Design review of the part built by this model. Coordinates are the model's own, in mm. A direction names the side the tool comes from. Coordinates: 2 decimals unless noted, no trailing zeros. Loops run counter-clockwise (first coordinate to the right, second up) from the corner with the lowest first, then second, coordinate; pieces in that order, holes last.
from build123d import *

# Parameters (mm, degrees)
F1_DEPTH = 130


with BuildPart() as f1:
    # F0 (on Front) → F1 (new body)
    with BuildSketch(Plane.XZ):
        with BuildLine():
            Line((-80.4885666445, 0), (-80.4885666445, -37.026398866))
            Line((-80.4885666445, -37.026398866), (80.4885666445, -37.026398866))
            Line((80.4885666445, -37.026398866), (80.4885666445, 37.026398866))
            ThreePointArc((80.4885666445, 37.026398866), (56.312606492, 15.964739969), (24.5885544515, 11.3112416162))
            ThreePointArc((24.5885544515, 11.3112416162), (23.4644064233, 5.2103284523), (20.0973115861, 0))
            ThreePointArc((20.0973115861, 0), (10.0486557931, -1.628361225), (0, 0))
            add(Edge.make_bspline(
                [(0, 0), (1.1070352702, -1.6801785988), (3.1184613885, -4.7329766513), (4.5940239288, -8.7749202813), (1.7421748157, -13.92092092), (0, -17.0645769686)],
                knots=[0, 0, 0, 0, 0.3226277316, 0.5861979859, 1, 1, 1, 1], degree=3))
            Line((0, -17.0645769686), (-68.7817037106, -17.0645769686))
            add(Edge.make_bspline(
                [(-69.5971027017, 0), (-68.7549732227, -1.0893751099), (-72.5978419161, -5.9254448151), (-70.4120398181, -12.0907470214), (-69.2717425761, -15.6012676406), (-68.7817037106, -17.0645769686)],
                knots=[0.3125236167, 0.3125236167, 0.3125236167, 0.3125236167, 0.5421460101, 0.7849492257, 1, 1, 1, 1], degree=3))
            Line((-69.5971027017, 0), (-80.4885666445, 0))
        make_face()
    extrude(amount=F1_DEPTH)


solid = f1.part
Q1. For line 1 (X direction, y = -21.5, z = -4.5); line 2 (Z direction, x = -50, y = -68.5); line 3 (Z direction, x = 31, y = -91.5), list the stretches that pass through material, from the lowest coordinate up.
Q2. The part is to be moulded in two halves that separate along X. For faces 1 (the cylindrical face through (56.73, -64.09, 16.16)), 2 (the flat face through (17, -130, -16)), 3 (the flat face through (-80.489, -64, -18)), 4 (the flat face through (80.489, -64, -1)), say which applies: pulls with the +X half, pulls with the -X half, needs draft (parallel to the pull), parting line crosses it, or undercut.
Q3. Machinability: for faces 5 (the flat face through (-1, -64, -37.026)), 6 (the flat face through (-34, -64, -17.065)), 7 (the flat face through (-75, -64, 0)), which of the approach directions +Z, -Z, +X, -X, +Y, -Y give a long, thin tool a straight path to every point of the face, cutting with its end or side? Answer none if there is none.
Q4. Clearance check with flat-ended pins moving along their axes: pin 1 Ø3.5 at (x, y) = (-77.5, -33) entering from +Z; pin 2 Ø5 at (x, y) = (11, -115.5) entering from +Z; pin 3 Ø20.5 at (x, y) = (-18, -81.5) entering from +Z. State where each tip first meets the part, or that it passes through.
Q5. Take a section at B-B, the plane z = 16. Write out the cut boundary in (x, y).
Q6. Take a section at A-A, the plane x = -62.5. Write out the cut boundary in (y, z), then the cut area to 3 significant figures.
Entries:
1. line 1: x = -80.49 to -70.82, 2.8 to 80.49
1. line 2: z = -37.03 to -17.06
1. line 3: z = -37.03 to 10.78
2. face 1: undercut
2. face 2: needs draft
2. face 3: pulls with the -X half
2. face 4: pulls with the +X half
3. face 5: -Z, +X, -X, +Y, -Y
3. face 6: +Z, +Y, -Y
3. face 7: +Z, -X, +Y, -Y
4. pin 1: stops at z = 0
4. pin 2: stops at z = -1.44
4. pin 3: stops at z = -17.06
5. outline: (56.39, -130) - (80.49, -130) - (80.49, 0) - (56.39, 0) - close
6. outline: (-130, -37.03) - (0, -37.03) - (0, -17.06) - (-130, -17.06) - close
6. area: 2,600 mm2
